The drawing under review shows one solid part. Ordinate dimensions are in mm from its lowest x, y, z. A direction names the side the tool comes from. Coordinates: 2 decimals unless noted, no trailing zeros. Loops run counter-clockwise (first coordinate to the right, second up) from the corner with the lowest first, then second, coordinate; pieces in that order, holes last. Notation, with made-up numbers: M 89.25,-39 L 121.25,-39 A22 cw 121.25,-10 Z; hole C 3.25,43 d5. An arc over 180 degrees is marked long. Put each result on its own line as item: value.
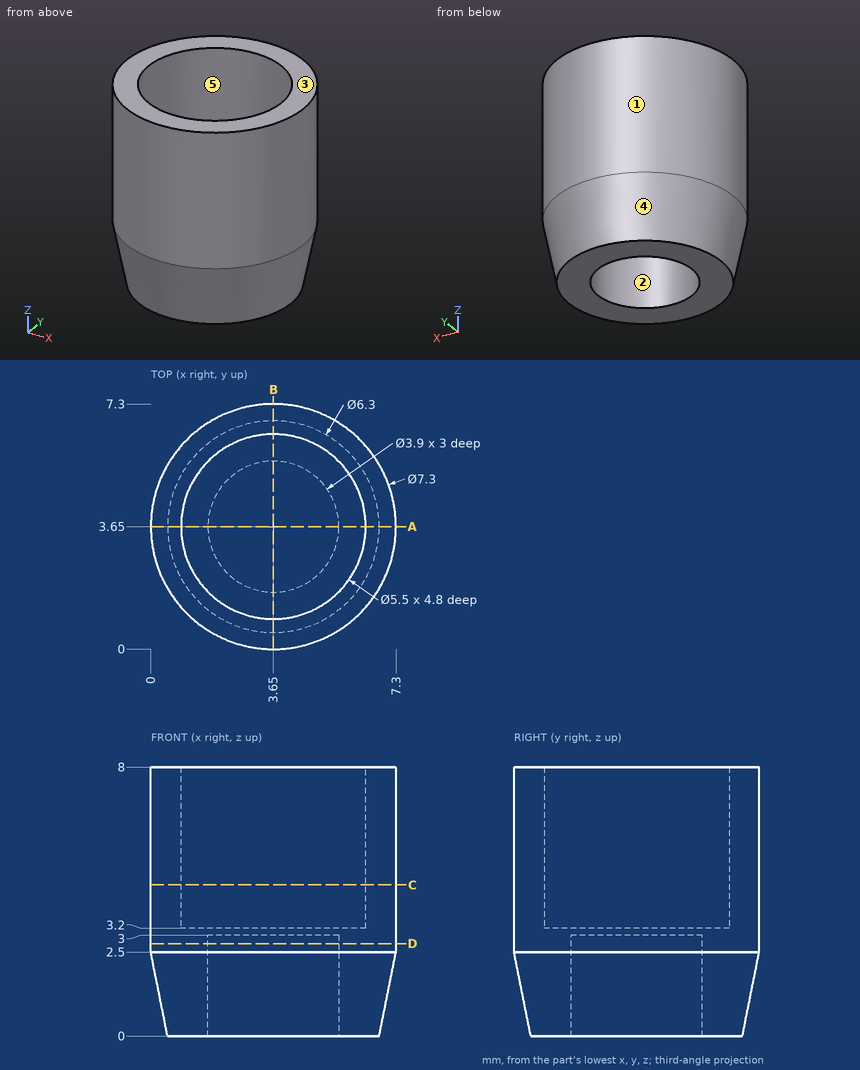
(1) Add section C-C (z = 4.5). Write out the cut boundary in (x, y).
Determined:
outline: C 3.65,3.65 d7.3; hole C 3.65,3.65 d5.5
(2) Add section D-D (z = 2.75). Write out the cut boundary in (x, y), plus the area to 3 significant figures.
Determined:
outline: C 3.65,3.65 d7.3; hole C 3.65,3.65 d3.9
area: 29.9 mm^2
(3) Draft analysis for pull direction Y (two halves, no side actions). For the marked faces 1, 2 and 3, state which applies: +Y half, -Y half, draft (parallel to the pull), parting line (faces both ways), or undercut.
Determined:
face 1: parting line
face 2: undercut
face 3: draft
(4) Tool access review of the marked faces 4 and 5: name each direction out of +Z, -Z, +X, -X, +Y, -Y from which nothing blocks a thin tool from reaching the whole face with its end or side.
Determined:
face 4: -Z
face 5: +Z
(5) Wall thickness on line 1 along Y through (x, z) = (3.65, 4.7); line 2 along Y through (x, z) = (4, 2.5): over which ranges is each line inside the solid? List them lowest first. Write a range as [from, to].
Determined:
line 1: y = [0, 0.9], [6.4, 7.3]
line 2: y = [0.02, 1.73], [5.57, 7.28]
(6) For pin 1 (1.5 mm diameter, centred on y = 2.5, z = 3, fed in from -X); pin 2 (3 mm diameter, centred on x = 1, z = 1.5, fed in from -Y); pin 3 (2 mm diameter, centred on x = 5, z = 4.5, fed in from +Y), all flat-tipped, find the tip position at first contact; note any pin that passes through.
Determined:
pin 1: stops at x = 0.02
pin 2: stops at y = 0.31
pin 3: stops at y = 7.28
(7) Add section A-A (y = 3.65). Write out the cut boundary in (x, z), plus the area to 4 significant figures.
Determined:
outline: M 0,2.5 L 0.5,0 L 1.7,0 L 1.7,3 L 5.6,3 L 5.6,0 L 6.8,0 L 7.3,2.5 L 7.3,8 L 6.4,8 L 6.4,3.2 L 0.9,3.2 L 0.9,8 L 0,8 Z
area: 19.05 mm^2
